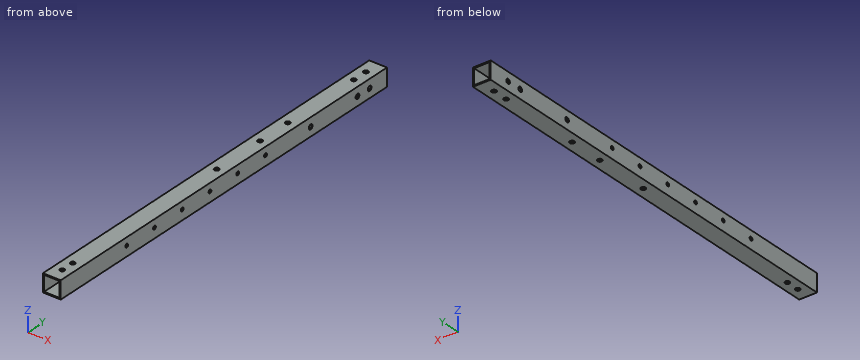
Autodesk Inventor part; units mm, degrees
ref_plane "YZ Plane" through (0, 0, 0) normal (1, 0, 0) x (0, 1, 0)
ref_plane "XZ Plane" through (0, 0, 0) normal (0, 1, 0) x (-1, 0, 0)
ref_plane "XY Plane" through (0, 0, 0) normal (0, 0, 1) x (1, 0, 0)
sketch "Sketch1" plane through (0, 0, 0) normal (0, 1, 0) x (-1, 0, 0)
  line L0 (0, 0) -> (-25.4, 0)
  line L1 (-25.4, 0) -> (-25.4, 25.4)
  line L2 (-25.4, 25.4) -> (0, 25.4)
  line L3 (0, 25.4) -> (0, 0)
  line L4 (-1.5875, 23.8125) -> (-23.8125, 23.8125)
  line L5 (-23.8125, 23.8125) -> (-23.8125, 1.5875)
  line L6 (-23.8125, 1.5875) -> (-1.5875, 1.5875)
  line L7 (-1.5875, 1.5875) -> (-1.5875, 23.8125)
  dimension "d0" = 25.4
  dimension "d2" = 25.4
  dimension "d3" = 1.5875
extrude "Extrusion1" add sketch "Sketch1" along normal blind 596.9
sketch "Sketch8" plane through (25.4, 0, 25.4) normal (1, 0, 0) x (0, 0, -1)
  circle A0 centre (12.7, 457.2) radius 3.3782
  circle A1 centre (11.1125, 374.65) radius 2.54
  circle A2 centre (11.1125, 323.85) radius 2.54
  circle A3 centre (11.1125, 273.05) radius 2.54
  circle A4 centre (11.1125, 222.25) radius 2.54
  circle A5 centre (11.1125, 171.45) radius 2.54
  circle A6 centre (11.1125, 120.65) radius 2.54
  circle A7 centre (12.7, 565.15) radius 3.3782
  circle A8 centre (12.7, 542.925) radius 3.3782
  line L0 (25.4, 0) -> (0, 0)
  line L1 (0, 596.9) -> (25.4, 596.9)
  line L2 (12.7, 596.9) -> (12.7, 0) construction
extrude "Extrusion7" cut sketch "Sketch8" against normal blind 25.4
sketch "Sketch9" plane through (25.4, 0, 0) normal (0, 0, -1) x (-1, 0, 0)
  circle A0 centre (12.7, 431.8) radius 3.3782
  line L0 (25.4, 440.055) -> (0, 440.055)
  line L1 (0, 368.3) -> (0, 440.055)
  line L2 (25.4, 368.3) -> (0, 368.3)
  line L3 (25.4, 440.055) -> (25.4, 368.3)
  circle A1 centre (12.7, 431.8) radius 3.3782
  circle A2 centre (12.7, 381) radius 3.3782
  circle A3 centre (12.7, 19.05) radius 3.302
  circle A4 centre (12.7, 38.1) radius 3.302
  arc A5 (3.175, 50.8) -> (0, 47.625) centre (3.175, 47.625) ccw
  line L4 (3.175, 50.8) -> (22.225, 50.8)
  arc A6 (25.4, 47.625) -> (22.225, 50.8) centre (22.225, 47.625) ccw
  line L5 (25.4, 47.625) -> (25.4, 4.445)
  line L6 (25.4, 4.445) -> (0, 4.445)
  line L7 (0, 47.625) -> (0, 4.445)
  circle A7 centre (12.7, 552.45) radius 3.3782
  circle A8 centre (12.7, 574.675) radius 3.3782
  circle A9 centre (12.7, 301.625) radius 3.3782
extrude "Extrusion8" cut sketch "Sketch9" against normal blind 25.4 contours A0 | A2 | A3 | A4 | A7 | A8 | A9
properties part number "Rebuild Edge Mount 2" material "Aluminum 6061"
Model file for the job. Use its own axes, mm. Give positions to 0.01 mm unless a question says otherwise; leave off trailing zeros. Write each loop counter-clockwise with the first axis right and the second up, starting at its lowest first coordinate (ties: lowest second). Pieces come first, ordered by that corner, then holes. Notation, with made-up numbers: (5.5, 52) - (18.5, 52) arc R20 cw to (18.5, 72) - close; hole circle Ø10 at (-15.5, 27). An arc over 180 degrees is marked (long way). One line per question, with ' | ' between items. Start each with the question number.
(1) Wall check: line 1 along Z through (x, y) = (24.55, 323.85); line 2 along X through (y, z) = (30, 3.25). Give the ranges that are in metal, low to high. Write a range as from..to.
(2) Pin check, flat tips, straight feed: P1, Ø12, axis at x = 16, y = 220, coming from the -Z side; P2, Ø6, axis at y = 542.925, z = 12.7, coming from the +X side. Stop position of each tip, or through.
(3) Slice it at A-A on y = 208. Write the cut outline in (x, z).
(4) Slice it at B-B on z = 5.5. Write the cut outline in (x, y).
Results below:
1) line 1: 0..11.75, 16.83..25.4 | line 2: 0..1.59, 23.81..25.4
2) P1: z = 0 | P2: through
3) outline: (0, 0) - (25.4, 0) - (25.4, 25.4) - (0, 25.4) - close; hole (1.59, 1.59) - (23.81, 1.59) - (23.81, 23.81) - (1.59, 23.81) - close
4) outline: (0, 0) - (1.59, 0) - (1.59, 596.9) - (0, 596.9) - close; (23.81, 0) - (25.4, 0) - (25.4, 596.9) - (23.81, 596.9) - close
